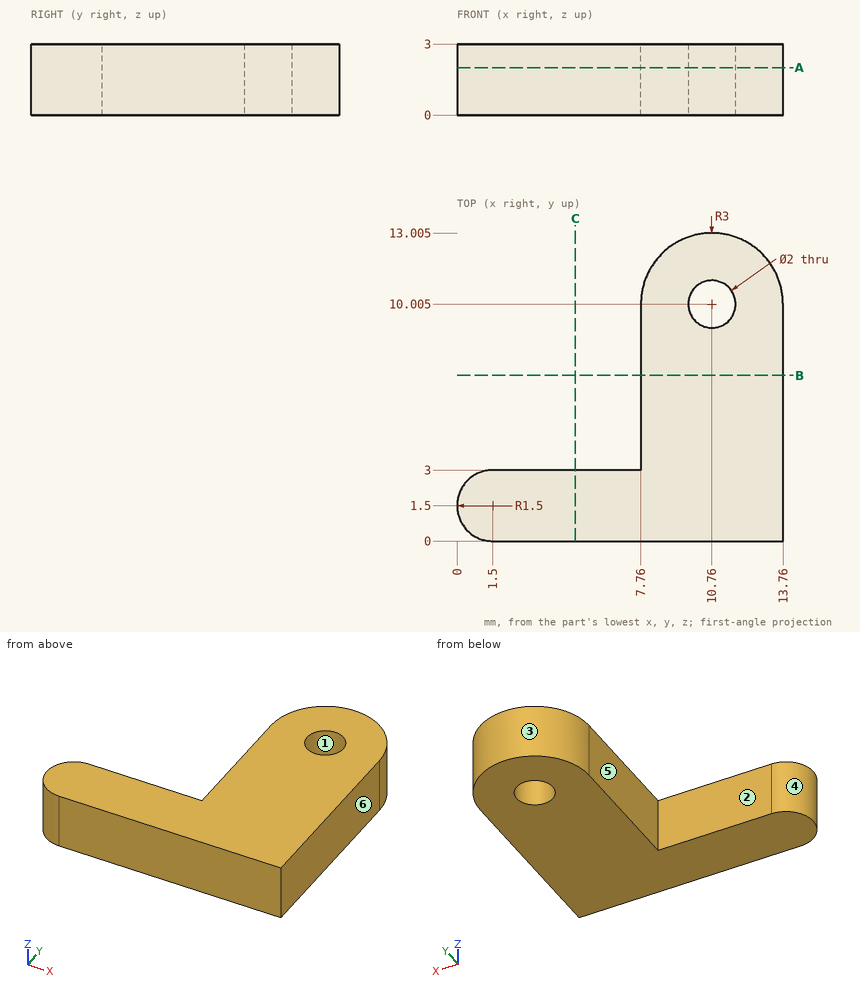
Study the drawing (mm; zero at the part's minimum x, y, z) and answer. A direction names the side the tool comes from. Give positions to 0.01 mm unless a question says otherwise; leave off trailing zeros. Write each loop counter-clockwise with the first axis right and the second up, starting at its lowest first coordinate (ties: lowest second). Pieces come first, ordered by that corner, then holes. Notation, with made-up numbers: (53, 45) -> (108, 45) arc R10 cw to (108, 52) -> close; hole circle Ø8 at (45.5, -17). An arc over 180 degrees is marked (long way). Answer as a JSON object with one key per item and string values. Group by question number.
1) The mould has two halves that part along X. Classify the marked faces 1, 2, 3 and 4: +X half, -X half, draft (parallel to the pull), parting line (faces both ways), or undercut.
2) A tool of negligible diameter and unlimited length cuts with its end or side. For the marked faces 5 and 6, from which of +Z, -Z, +X, -X, +Y, -Y can it reach the whole face along a straight path? Write none if from no direction.
3) Find section A-A (z = 2). Write down the section's boundary in (x, y) (1 decimal).
4) Find section C-C (x = 5). Write down the section's boundary in (y, z).
5) Find section B-B (y = 7). Write down the section's boundary in (x, z).
6) Consider L1, parallel to Y at x = 4, z = 1.6; L2, parallel to X at y = 5.75, z = 0.35; L3, parallel to Y at x = 12.75, z = 2.6. Determine where each line is inside the solid, lowest interval first. Write a range as from..to.
Values follow:
{
 "1": {"face 1": "undercut", "face 2": "draft", "face 3": "parting line", "face 4": "-X half"},
 "2": {"face 5": "+Z, -Z, -X, +Y", "face 6": "+Z, -Z, +X, +Y, -Y"},
 "3": {"outline": "(1.5, 0) -> (13.8, 0) -> (13.8, 10) arc R3 ccw to (7.8, 10) -> (7.8, 3) -> (1.5, 3) arc R1.5 ccw to start; hole circle Ø2 at (10.8, 10)"},
 "4": {"outline": "(0, 0) -> (3, 0) -> (3, 3) -> (0, 3) -> close"},
 "5": {"outline": "(7.76, 0) -> (13.76, 0) -> (13.76, 3) -> (7.76, 3) -> close"},
 "6": {"L1": "y = 0..3", "L2": "x = 7.76..13.76", "L3": "y = 0..12.25"}
}
